Job drawing, mm, ordinate dimensions from the low corner. One solid piece. A direction names the side the tool comes from. Give positions to 0.01 mm unless a question says otherwise; leave off trailing zeros. Order: outer loops, then holes, each group sorted by start corner. A loop starts at its lowest first (then second) coordinate and runs counter-clockwise, first axis right, second up. Notation, with made-up numbers: (-24.5, -36) - (-0.5, -36) arc R16 cw to (-0.5, -16) - close; hole circle Ø11 at (52, 72.5). An arc over 180 degrees is marked (long way). One line per item, written item: value.
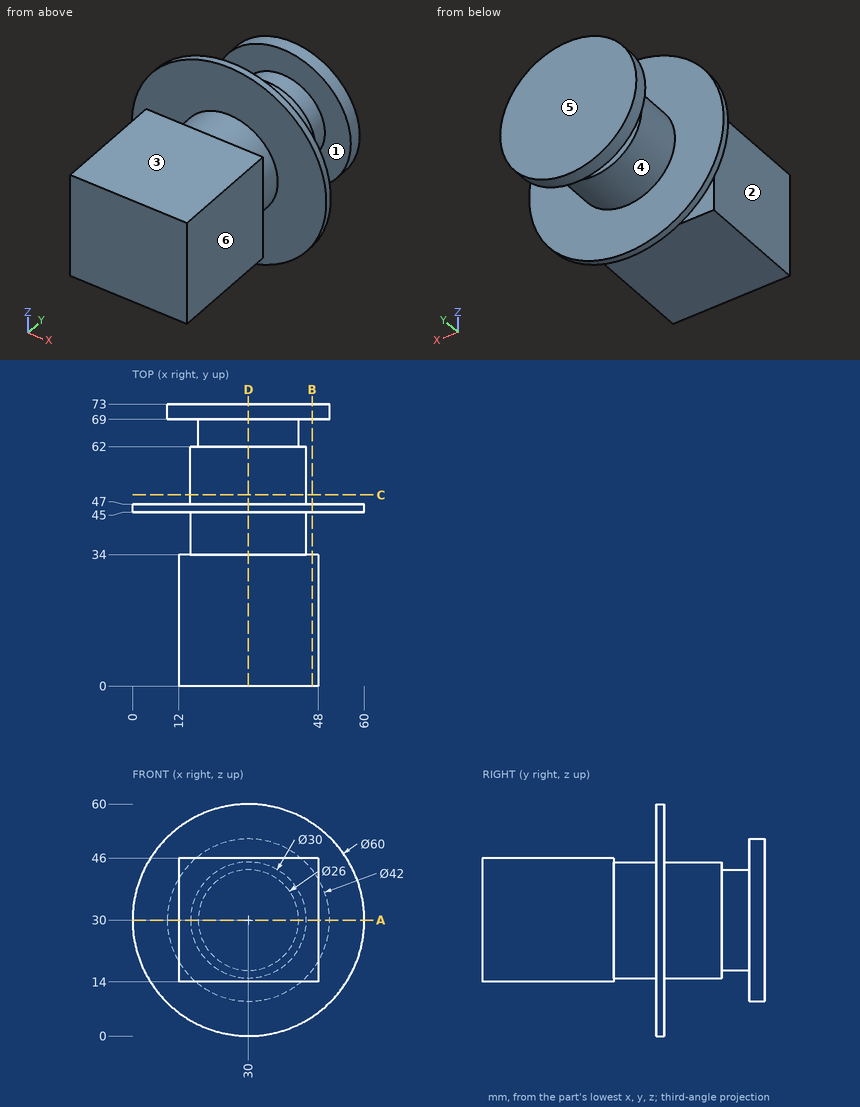
1) Slice it at C-C on y = 49.5. Write the cut outline in (x, z).
Answer:
outline: circle Ø30 at (30, 30)
2) Drop flat-ended pins along their axis: P1, Ø10, axis at x = 25, y = 18.5, coming from the +Z side; P2, Ø10, axis at x = 52.5, y = 49.5, coming from the +Z side; P3, Ø4, axis at x = 13, z = 6.5, coming from the -Y side. Give the stop position or say it passes through.
Answer:
P1: stops at z = 46
P2: stops at z = 53.87
P3: stops at y = 45
3) Slice it at A-A on z = 30. Write the cut outline in (x, y).
Answer:
outline: (0, 45) - (15, 45) - (15, 34) - (12, 34) - (12, 0) - (48, 0) - (48, 34) - (45, 34) - (45, 45) - (60, 45) - (60, 47) - (45, 47) - (45, 62) - (43, 62) - (43, 69) - (51, 69) - (51, 73) - (9, 73) - (9, 69) - (17, 69) - (17, 62) - (15, 62) - (15, 47) - (0, 47) - close
4) Two-plate mould, pull along Y, no slides. Class the marked faces 4, 5 and 6: pulls with the +Y half, pulls with the -Y half, needs draft (parallel to the pull), parting line crosses it, or undercut.
Answer:
face 4: undercut
face 5: pulls with the +Y half
face 6: needs draft
5) Slice it at D-D on x = 30. Write the cut outline in (y, z).
Answer:
outline: (0, 14) - (34, 14) - (34, 15) - (45, 15) - (45, 0) - (47, 0) - (47, 15) - (62, 15) - (62, 17) - (69, 17) - (69, 9) - (73, 9) - (73, 51) - (69, 51) - (69, 43) - (62, 43) - (62, 45) - (47, 45) - (47, 60) - (45, 60) - (45, 45) - (34, 45) - (34, 46) - (0, 46) - close
6) Which spindle directions (+Z, -Z, +X, -X, +Y, -Y) get a long thin tool onto all of the face, cutting with end or side? Do the marked faces 1, 2 and 3. Say none if no direction does.
Answer:
face 1: none
face 2: +Z, -Z, -X, -Y
face 3: +Z, +X, -X, -Y
7) Slice it at B-B on x = 46.5. Write the cut outline in (y, z), then the cut area to 3 significant figures.
Answer:
outline: (0, 14) - (34, 14) - (34, 46) - (0, 46) - close; (45, 4.95) - (47, 4.95) - (47, 55.05) - (45, 55.05) - close; (69, 17.01) - (73, 17.01) - (73, 42.99) - (69, 42.99) - close
area: 1,290 mm2
8) Wall check: line 1 along Y through (x, z) = (35, 47.5); line 2 along Z through (x, y) = (25, 9); line 3 along X through (y, z) = (25.5, 20). Give the ranges that are in metal, low to high. Write a range as [from, to].
Answer:
line 1: y = [45, 47], [69, 73]
line 2: z = [14, 46]
line 3: x = [12, 48]
